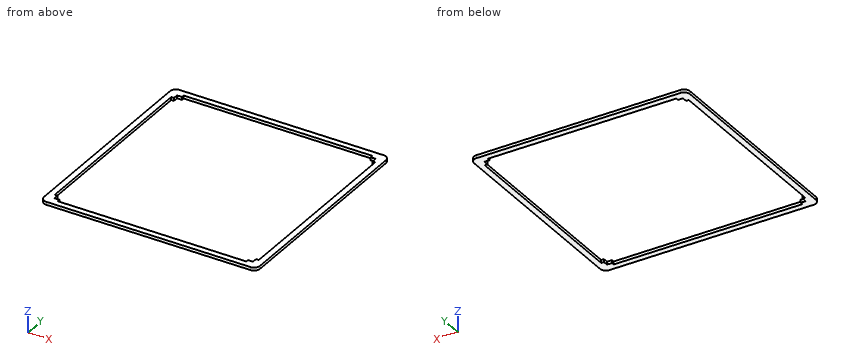
```python
from build123d import *

# Parameters (mm, degrees)
EXTRUDE_1_DEPTH = 3


with BuildPart() as part:
    # 草图1 → 凸台-拉伸1 (new body)
    with BuildSketch(Plane.XY):
        with BuildLine():
            Line((-8.75, 202.75), (-8.75, -2.75))
            ThreePointArc((-8.75, -2.75), (-6.992640687, -6.992640687), (-2.75, -8.75))
            Line((-2.75, -8.75), (202.75, -8.75))
            ThreePointArc((202.75, -8.75), (206.992640687, -6.992640687), (208.75, -2.75))
            Line((208.75, -2.75), (208.75, 202.75))
            ThreePointArc((208.75, 202.75), (206.992640687, 206.992640687), (202.75, 208.75))
            Line((202.75, 208.75), (-2.75, 208.75))
            ThreePointArc((-2.75, 208.75), (-6.992640687, 206.992640687), (-8.75, 202.75))
        make_face()
        Polygon((5, 202.75), (5, 200), (0, 200), (0, 195), (-2.75, 195), (-2.75, 5), (0, 5), (0, 0), (5, 0), (5, -2.75), (195, -2.75), (195, 0), (200, 0), (200, 5), (202.75, 5), (202.75, 195), (200, 195), (200, 200), (195, 200), (195, 202.75), align=None, mode=Mode.SUBTRACT)
    extrude(amount=EXTRUDE_1_DEPTH)


solid = part.part
```
Input: part model. Units: mm. Frame: model coordinates. Round coordinates to 2 decimals unless told otherwise and drop trailing zeros. Write each loop counter-clockwise with the first axis right and the second up, starting at its lowest first coordinate (ties: lowest second). Pieces come first, ordered by that corner, then holes. Notation, with made-up numbers: (0, 62.25) -> (53, 62.25) arc R22 cw to (53, 101.25) -> close; hole circle Ø4 at (26, 4). An arc over 180 degrees is marked (long way). Answer as CSV lines item,"result".
1. Section B-B (z = 1.6). Return the cut outline in (x, y), plus the area to 3 significant figures.
Geometry says:
outline,"(-8.75, -2.75) arc R6 ccw to (-2.75, -8.75) -> (202.75, -8.75) arc R6 ccw to (208.75, -2.75) -> (208.75, 202.75) arc R6 ccw to (202.75, 208.75) -> (-2.75, 208.75) arc R6 ccw to (-8.75, 202.75) -> close; hole (-2.75, 5) -> (0, 5) -> (0, 0) -> (5, 0) -> (5, -2.75) -> (195, -2.75) -> (195, 0) -> (200, 0) -> (200, 5) -> (202.75, 5) -> (202.75, 195) -> (200, 195) -> (200, 200) -> (195, 200) -> (195, 202.75) -> (5, 202.75) -> (5, 200) -> (0, 200) -> (0, 195) -> (-2.75, 195) -> close"
area,"5,190 mm^2"
2. Section A-A (x = 140). Return the cut outline in (y, z), plus the area to 3 significant figures.
Geometry says:
outline,"(-8.75, 0) -> (-2.75, 0) -> (-2.75, 3) -> (-8.75, 3) -> close; (202.75, 0) -> (208.75, 0) -> (208.75, 3) -> (202.75, 3) -> close"
area,"36.0 mm^2"
3. Ray query, L1, parallel to Y at x = 53, z = 1.2; L2, parallel to X at y = 2.5, z = 2.2. Return the intervals inside material, ascending. Write a range as [from, to].
Geometry says:
L1,"y = [-8.75, -2.75], [202.75, 208.75]"
L2,"x = [-8.75, 0], [200, 208.75]"
